Autodesk Inventor part; units mm, degrees
ref_plane "YZ Plane" through (0, 0, 0) normal (1, 0, 0) x (0, 1, 0)
ref_plane "XZ Plane" through (0, 0, 0) normal (0, 1, 0) x (-1, 0, 0)
ref_plane "XY Plane" through (0, 0, 0) normal (0, 0, 1) x (1, 0, 0)
sketch "Skizze1" plane through (0, 0, 0) normal (0, 0, 1) x (1, 0, 0)
  line L0 (-8, -5.5) -> (8, -5.5)
  line L1 (8, -5.5) -> (8, 5.5)
  line L2 (8, 5.5) -> (-8, 5.5)
  line L3 (-8, 5.5) -> (-8, -5.5)
  line L4 (-8, -5.5) -> (8, 5.5) construction
  line L5 (8, -5.5) -> (-8, 5.5) construction
  circle A0 centre (0, 0) radius 5.5
  circle A1 centre (0, 0) radius 4
  dimension "d0" = 11
  dimension "d1" = 16
  dimension "d6" = 8
extrude "Extrusion1" add sketch "Skizze1" along normal blind 5 contours L3 L2 A0 L0 | A0 L2 L1 L0
extrude "Extrusion2" add sketch "Skizze1" against normal blind 1 contours L3 L2 A0 L0 | A0 L2 L1 L0 | A0 | A1
extrude "Extrusion3" cut sketch "Skizze1" against normal through all contours A1
properties part number "rotSpanner" material "ABS-Kunststoff"
CAD build for the part. Positions are in the model's coordinates, mm. A direction names the side the tool comes from. Coordinates: 2 decimals unless noted, no trailing zeros. Order: outer loops, then holes, each group sorted by start corner. A loop starts at its lowest first (then second) coordinate and runs counter-clockwise, first axis right, second up.
(1) Drill centre lines: L1, parallel to Y at x = 0, z = -0.3; L2, parallel to Z at x = -1.5, y = -4; L3, parallel to X at y = 2.5, z = 0.9. Where is each one in solid material? Low to high.
Solution:
L1: y = -5.5 to -4, 4 to 5.5
L2: z = -1 to 0
L3: x = -8 to -4.9, 4.9 to 8
(2) Which spindle directions (+Z, -Z, +X, -X, +Y, -Y) get a long thin tool onto all of the face, cutting with end or side? Do faces 4 (the face through (-2, 4, -1)), 5 (the face through (-5.5, -0.1, 2.5)). Say none if no direction does.
Solution:
face 4: -Z, +X, -X, +Y, -Y
face 5: +Z
(3) Saw through at C-C, the plane x = -2.25. Write the cut outline in (y, z).
Solution:
outline: (-5.5, -1) - (-3.31, -1) - (-3.31, 0) - (-5.02, 0) - (-5.02, 5) - (-5.5, 5) - close; (3.31, -1) - (5.5, -1) - (5.5, 5) - (5.02, 5) - (5.02, 0) - (3.31, 0) - close
(4) Saw through at A-A, the plane y = 0. Write the cut outline in (x, z).
Solution:
outline: (-8, -1) - (-4, -1) - (-4, 0) - (-5.5, 0) - (-5.5, 5) - (-8, 5) - close; (4, -1) - (8, -1) - (8, 5) - (5.5, 5) - (5.5, 0) - (4, 0) - close
(5) Saw through at D-D, the plane x = -5. Write the cut outline in (y, z), and give its area (3 significant figures).
Solution:
outline: (-5.5, -1) - (5.5, -1) - (5.5, 5) - (2.29, 5) - (2.29, 0) - (-2.29, 0) - (-2.29, 5) - (-5.5, 5) - close
area: 43.1 mm2
(6) Mould opens along Y. For faces 1 (the face through (-6, 0, 5)), 2 (the face through (-4, -2, 0)), 3 (the face through (5.5, 0.1, 2.5)) say: released by +Y, released by -Y, zero draft, split by the parting line, or undercut.
Solution:
face 1: zero draft
face 2: undercut
face 3: undercut
